from build123d import *

# Parameters (mm, degrees)
SKETCH1_W                = 50.8
SKETCH1_H                = 44.45
BOSS_EXTRUDE1_DEPTH      = 2.3876
F_0_257_DIAMETER_HOLE1_D = 6.5278
FILLET1_R                = 12.7


with BuildPart() as part:
    # Sketch1 → Boss-Extrude1 (new body, symmetric)
    with BuildSketch(Plane.XY):
        with Locations((0, 22.225)):
            Rectangle(SKETCH1_W, SKETCH1_H)
    extrude(amount=BOSS_EXTRUDE1_DEPTH, both=True)

    # F (0.257) Diameter Hole1 (through all)
    with Locations(Plane.XY.offset(2.3876)):
        with Locations((-17.4625, 12.4968), (17.4625, 12.4968)):
            Hole(F_0_257_DIAMETER_HOLE1_D / 2)

    # Fillet1
    fillet1_edges = [part.edges().sort_by_distance(p)[0] for p in [
        (-25.4, 44.45, 0),
        (25.4, 44.45, 0),
    ]]
    fillet(fillet1_edges, radius=FILLET1_R)


solid = part.part
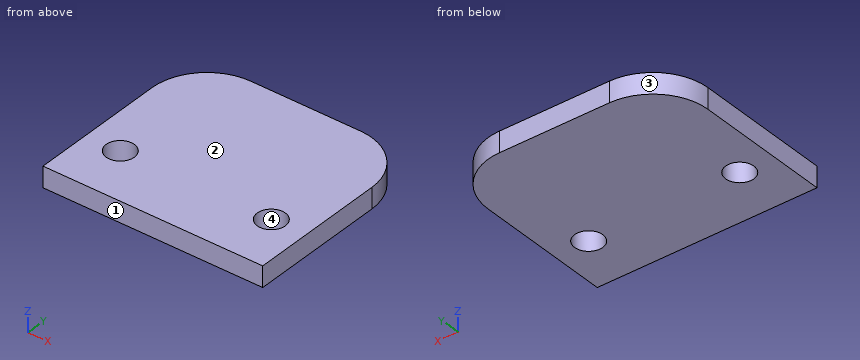
Design review of the part built by this model. Coordinates are the model's own, in mm. Face numbers are marked on the shaded views. Round coordinates to 2 decimals unless told otherwise and drop trailing zeros. Loops run counter-clockwise (first coordinate to the right, second up) from the corner with the lowest first, then second, coordinate; pieces in that order, holes last. Notation, with made-up numbers: (49.5, 36) - (85.5, 36) arc R26 ccw to (85.5, 56) - close; hole circle Ø5 at (-9.5, 58.5). An arc over 180 degrees is marked (long way). One line per item, written item: value. Start each with the question number.
1) To check wall thickness, follow L1, parallel to Y at x = 16, z = 0.5; L2, parallel to X at y = 15.5, z = 1.7; L3, parallel to Y at x = -18, z = 1.2. State the ranges of each line that lie inside material, in increasing order. Write a range as from..to.
2) Consider section C-C on z = -1.2. Give the boundary of the cut face in (x, y), then the cut area to 3 significant figures.
3) Consider section A-A on y = 14. Give the boundary of the cut face in (x, z).
4) Consider section B-B on x = -16. Give the boundary of the cut face in (y, z), then the cut area to 3 significant figures.
5) Draft analysis for pull direction Y (two halves, no side actions). For the marked faces 1, 2, 3 and 4, state which applies: +Y half, -Y half, draft (parallel to the pull), parting line (faces both ways), or undercut.
6) Consider section D-D on x = 18. Give the boundary of the cut face in (y, z), then the cut area to 3 significant figures.
Reported:
1. L1: y = 0..9.58, 15.41..44.01
1. L2: x = -25.4..-18.74, -16.18..16.18, 18.74..25.4
1. L3: y = 0..9.28, 15.72..43.29
2. outline: (-25.4, 0) - (25.4, 0) - (25.4, 31.75) arc R12.7 ccw to (12.7, 44.45) - (-12.7, 44.45) arc R12.7 ccw to (-25.4, 31.75) - close; hole circle Ø6.53 at (-17.46, 12.5); hole circle Ø6.53 at (17.46, 12.5)
2. area: 2,120 mm^2
3. outline: (-25.4, -2.39) - (-20.36, -2.39) - (-20.36, 2.39) - (-25.4, 2.39) - close; (-14.57, -2.39) - (14.57, -2.39) - (14.57, 2.39) - (-14.57, 2.39) - close; (20.36, -2.39) - (25.4, -2.39) - (25.4, 2.39) - (20.36, 2.39) - close
4. outline: (0, -2.39) - (9.58, -2.39) - (9.58, 2.39) - (0, 2.39) - close; (15.41, -2.39) - (44.01, -2.39) - (44.01, 2.39) - (15.41, 2.39) - close
4. area: 182 mm^2
5. face 1: -Y half
5. face 2: draft
5. face 3: +Y half
5. face 4: undercut
6. outline: (0, -2.39) - (9.28, -2.39) - (9.28, 2.39) - (0, 2.39) - close; (15.72, -2.39) - (43.29, -2.39) - (43.29, 2.39) - (15.72, 2.39) - close
6. area: 176 mm^2
